Autodesk Inventor part; units mm, degrees
ref_plane "YZ Plane" through (0, 0, 0) normal (1, 0, 0) x (0, 1, 0)
ref_plane "XZ Plane" through (0, 0, 0) normal (0, 1, 0) x (-1, 0, 0)
ref_plane "XY Plane" through (0, 0, 0) normal (0, 0, 1) x (1, 0, 0)
sketch "Sketch1" plane through (0, 0, 0) normal (0, 0, 1) x (1, 0, 0)
  line L0 (-44.45, -44.323) -> (44.45, -44.323)
  line L1 (44.45, -44.323) -> (44.45, 44.323)
  line L2 (44.45, 44.323) -> (-44.45, 44.323)
  line L3 (-44.45, 44.323) -> (-44.45, -44.323)
  line L4 (-44.45, -44.323) -> (44.45, 44.323) construction
  line L5 (44.45, -44.323) -> (-44.45, 44.323) construction
  point P0 (0, 0)
  dimension "d0" = 88.9
  dimension "d1" = 88.646
extrude "Extrusion1" add sketch "Sketch1" along normal blind 2.159
sketch "Sketch3" plane through (-44.45, 44.323, 0) normal (0, 1, 0) x (1, 0, 0)
  circle A0 centre (44.45, 0) radius 2.9972
  dimension "d4" = 5.9944
extrude "Extrusion2" add sketch "Sketch3" along normal blind 1.27 and the other way blind 88.773
sketch "Sketch4" plane through (0, 0, 2.159) normal (0, 0, 1) x (1, 0, 0)
  circle A0 centre (-27.1018, 35.7124) radius 2.1828
  line L0 (-44.45, 44.323) -> (-44.45, -44.323)
  line L1 (-2.0789, 44.323) -> (-44.45, 44.323)
  line L2 (-44.45, 0) -> (0, 0)
  circle A1 centre (-27.1018, -35.7124) radius 2.1828
  line L3 (-2.9972, -44.45) -> (2.9972, -44.45)
  line L4 (0, -44.45) -> (0, 45.593)
  line L5 (2.9972, 45.593) -> (-2.9972, 45.593)
  circle A2 centre (27.1018, 35.7124) radius 2.1828
  circle A3 centre (27.1018, -35.7124) radius 2.1828
  dimension "d9" = 17.3482
  dimension "d10" = 4.3656
  dimension "d11" = 8.6106
extrude "Extrusion3" add sketch "Sketch4" along normal blind 15 and the other way blind 5
properties part number "Hinge"
CAD build for the part. Positions are in the model's coordinates, mm. A direction names the side the tool comes from. Round coordinates to 2 decimals unless told otherwise and drop trailing zeros. Loops run counter-clockwise (first coordinate to the right, second up) from the corner with the lowest first, then second, coordinate; pieces in that order, holes last. Notation, with made-up numbers: M 56,78.25 L 99,78.25 A17 cw 99,85.25 Z; hole C 67,68 d2. An arc over 180 degrees is marked long. Return JSON: item names as keys, results as strings. Group by question number.
(1) Mould opens along X. For faces 5 (the cylindrical face through (-27.386, -37.877, 9.554)), 6 (the cylindrical face through (25.49, 34.24, 9.55)), 7 (the flat face through (44.45, -1, 1)), 8 (the flat face through (-27, -36, 17.159)) say: +X half, -X half, draft (parallel to the pull), parting line (faces both ways), or undercut.
(2) Saw through at C-C, the plane x = 0. List the corners of the cut face in (y, z).
(3) Wall check: probe 1 along Z at (x, y) = (-17, 13.5); probe 2 along Y at (x, z) = (-25.5, 14); probe 3 along Z at (x, y) = (0.5, 17.5). Give the ranges that are in metal, low to high. Write a range as [from, to].
(4) Tool access for faces 1 (the cylindrical face through (-29.282, -35.616, -1.401)), 2 (the cylindrical face through (-29.282, 35.616, 9.554)), 3 (the flat face through (-27, -36, -2.841)), 4 (the flat face through (27, -36, -2.841)): list every direction of +Z, -Z, +X, -X, +Y, -Y with a clear straight run to the whole face (end or side of a thin tool).
(5) Saw through at A-A, the plane y = -10.5. List the corners of the cut face in (x, z).
(6) Drop flat-ended pins along their axis: P1, Ø3.5, axis at x = 27.5, y = -35, coming from the -Z side; P2, Ø10, axis at x = -21.5, z = 10, coming from the +Y side; P3, Ø1.7, axis at x = -27.5, z = 1.5, coming from the +Y side; P4, Ø1.5, axis at x = -22.5, z = 5.5, coming from the -Y side. Give the stop position or say it passes through.
(7) Saw through at B-B, the plane z = 4.75. List the corners of the cut face in (x, y), and give its area (3 significant figures).
Answer list:
{
 "1": {"face 5": "undercut", "face 6": "undercut", "face 7": "+X half", "face 8": "draft"},
 "2": {"outline": "M -44.45,-3 L 45.59,-3 L 45.59,3 L -44.45,3 Z"},
 "3": {"probe 1": "[0, 2.16]", "probe 2": "[-37.2, -34.23], [34.23, 37.2]", "probe 3": "[-2.96, 2.96]"},
 "4": {"face 1": "-Z", "face 2": "+Z", "face 3": "-Z, -X, +Y, -Y", "face 4": "-Z, +X, +Y, -Y"},
 "5": {"outline": "M -44.45,0 L -3,0 A3 ccw 3,0 L 44.45,0 L 44.45,2.16 L 2.08,2.16 A3 ccw -2.08,2.16 L -44.45,2.16 Z"},
 "6": {"P1": "z = -2.84", "P2": "y = 37.81", "P3": "y = 44.32", "P4": "through"},
 "7": {"outline": "C -27.1,-35.71 d4.37; C -27.1,35.71 d4.37; C 27.1,-35.71 d4.37; C 27.1,35.71 d4.37", "area": "59.9 mm2"}
}
